Could you check a few things on this model? Use its own coordinates, in mm. A direction names the side the tool comes from. Give positions to 0.01 mm unless a question says otherwise; leave off trailing zeros. Order: outer loops, then holes, each group sorted by start corner. A loop starts at its lowest first (then second) coordinate and runs counter-clockwise, first axis right, second up.
(1) Imagine slicing it at B-B, the plane x = 10. Write out the boundary of the cut face in (y, z), then the cut area to 3 significant figures.
(2) If we mould it in two halves opening along Z, with no side actions, what happens to faces 3 (the flat face through (7, 2, -86.169)), 4 (the flat face through (-12.881, 2, 0)), 5 (the cylindrical face through (7.091, 11.9, -71.314)), 6 (the flat face through (7, 2, 9.831))? For each: released by +Z, released by -Z, zero draft, split by the parting line, or undercut.
(3) If I drill on probe 1 along Z at (x, y) = (7, 11.5); probe 2 along Y at (x, z) = (21.5, -10); probe 3 along Z at (x, y) = (19.5, 2.5), over which ranges is the centre line in solid material (lowest first)?
(4) On a 3-axis mill with a long thin cutter (end or side, diameter ignored), from which of +Z, -Z, +X, -X, +Y, -Y can I reach the whole of each face in a straight line? I mean faces 1 (the cylindrical face through (8.706, 0.783, -34.819)), 2 (the cylindrical face through (7.091, -8.6, -71.314)). Say none if no direction works.
(5) Imagine slicing it at A-A, the plane y = 7. Write out the boundary of the cut face in (x, z), then the cut area to 3 significant figures.
(6) Will these pins go through, and if not, where does the flat tip stop? pin 1 (12 mm diameter, centred on x = 19.5, z = -15, fed in from -Y); pin 2 (1.2 mm diameter, centred on x = 20, y = 3, fed in from -Z); pin 3 (2 mm diameter, centred on x = 6.5, y = -4, fed in from +Z).
from build123d import *

# Parameters (mm, degrees)
SKETCH1_W           = 40
SKETCH1_H           = 20
BOSS_EXTRUDE1_DEPTH = 4
SKETCH3_R           = 2
BOSS_EXTRUDE3_DEPTH = 50
SKETCH5_W           = 26
SKETCH5_H           = 13.5
BOSS_EXTRUDE4_DEPTH = 2
BOSS_EXTRUDE5_DEPTH = 2
SKETCH7_R           = 1.25
CUT_EXTRUDE1_DEPTH  = 23


with BuildPart() as part:
    # Sketch1 → Boss-Extrude1 (new body)
    with BuildSketch(Plane(origin=(0, 0, 0), x_dir=(1, 0, 0), z_dir=(0, 1, 0))):
        with Locations((7.118644068, 0.169491525)):
            Rectangle(SKETCH1_W, SKETCH1_H)
    extrude(amount=BOSS_EXTRUDE1_DEPTH)

    # Sketch3 → Boss-Extrude3 (add)
    with BuildSketch(Plane(origin=(0, 0, -10.169491525), x_dir=(-1, 0, 0), z_dir=(0, 0, -1))):
        with Locations((-7.118644068, 2)):
            Circle(SKETCH3_R)
    extrude(amount=BOSS_EXTRUDE3_DEPTH)

    # Sketch5 → Boss-Extrude4 (add)
    with BuildSketch(Plane(origin=(7.118644068, 0, 0), x_dir=(0, 0, -1), z_dir=(1, 0, 0))):
        with Locations((73.169491525, 8.75)):
            Rectangle(SKETCH5_W, SKETCH5_H)
        with Locations((73.169491525, -4.75)):
            Rectangle(SKETCH5_W, SKETCH5_H)
    extrude(amount=BOSS_EXTRUDE4_DEPTH)

    # Sketch6 → Boss-Extrude5 (add)
    with BuildSketch(Plane.ZY.offset(-7.118644068)):
        Polygon((-60.169491525, -11.5), (-60.169491525, 0), (-60.169491525, 4), (-60.169491525, 15.5), (-86.169491525, 15.5), (-86.169491525, -11.5), align=None)
    extrude(amount=BOSS_EXTRUDE5_DEPTH)

    # Sketch7 → Cut-Extrude1 (cut, through all)
    with BuildSketch(Plane.ZY.offset(-5.118644068)):
        with Locations((-83.564955349, -8.654979701)):
            Circle(SKETCH7_R)
        with Locations((-70.064955349, 11.845020299)):
            Circle(SKETCH7_R)
        with Locations((-70.064955349, -8.654979701)):
            Circle(SKETCH7_R)
        with Locations((-83.564955349, 11.845020299)):
            Circle(SKETCH7_R)
    extrude(amount=-CUT_EXTRUDE1_DEPTH, mode=Mode.SUBTRACT)


solid = part.part
Answer block:
1. outline: (0, -10.17) - (4, -10.17) - (4, 9.83) - (0, 9.83) - close
1. area: 80.0 mm2
2. face 3: released by -Z
2. face 4: zero draft
2. face 5: undercut
2. face 6: released by +Z
3. probe 1: z = -86.17 to -84.77, -82.36 to -71.27, -68.86 to -60.17
3. probe 2: y = 0 to 4
3. probe 3: z = -10.17 to 9.83
4. face 1: none
4. face 2: +X, -X
5. outline: (5.12, -86.17) - (9.12, -86.17) - (9.12, -60.17) - (5.12, -60.17) - close
5. area: 104 mm2
6. pin 1: stops at y = 0
6. pin 2: stops at z = -10.17
6. pin 3: stops at z = -60.17
